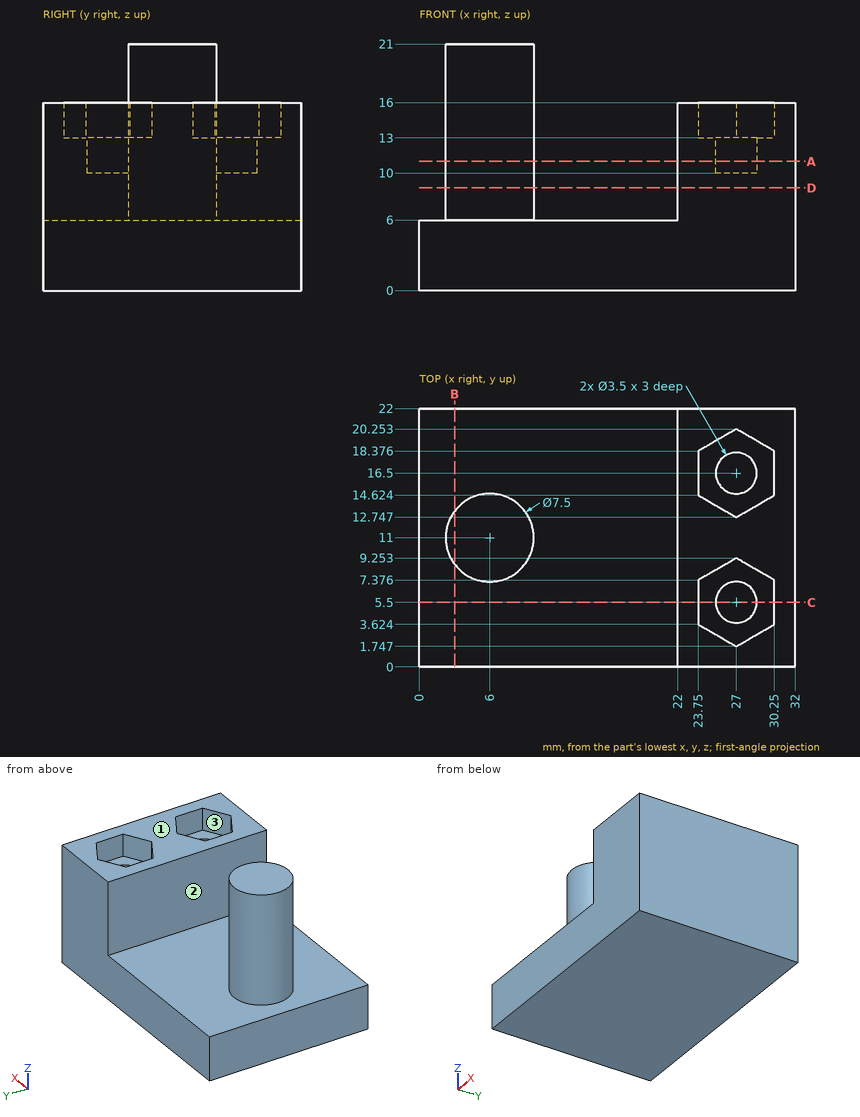
Geometry: see drawing. Coordinates: mm, zero at the bounding-box minimum. A direction names the side the tool comes from. Give positions to 0.01 mm unless a question says otherwise; leave off trailing zeros. Loops run counter-clockwise (first coordinate to the right, second up) from the corner with the lowest first, then second, coordinate; pieces in that order, holes last. Notation, with made-up numbers: (-8.75, 23.5) - (11.25, 23.5) arc R19 ccw to (11.25, 54.5) - close; hole circle Ø11 at (75.25, 71). An arc over 180 degrees is marked (long way). One line per question, with ' | ' between items. Start each with the question number.
(1) Section query D-D on z = 8.75. Return loops of the section in (x, y), then the cut area to 3 significant figures.
(2) Section query C-C on y = 5.5. Return loops of the section in (x, z), then the cut area to 3 significant figures.
(3) Contact query for flat-ended pins moving along their axis: pin 1 (3 mm diameter, centred on y = 12, z = 9.5, fed in from -X); pin 2 (4 mm diameter, centred on x = 27, y = 17, fed in from +Z); pin 3 (12 mm diameter, centred on x = 25.5, z = 15.5, fed in from -Y); pin 4 (8 mm diameter, centred on x = 26, y = 13.5, fed in from +Z). Output: stop coordinate, or through.
(4) Ray query, line 1 (Y direction, x = 27, z = 12.2); line 2 (X direction, y = 8, z = 15.25); line 3 (Z direction, x = 7.5, y = 5.25). Return the intervals inside material, ascending. Write a range as from..to.
(5) Section query A-A on z = 11. Return loops of the section in (x, y), then the cut area to 3 significant figures.
(6) Section query B-B on x = 3. Return loops of the section in (y, z).
(7) Reachability of the marked faces 1, 2 and 3 from +Z, -Z, +X, -X, +Y, -Y: full face, straight path, thin tool, end or side. Return the list, or none.
The answers:
1) outline: circle Ø7.5 at (6, 11); (22, 0) - (32, 0) - (32, 22) - (22, 22) - close | area: 264 mm2
2) outline: (0, 0) - (32, 0) - (32, 16) - (30.25, 16) - (30.25, 13) - (28.75, 13) - (28.75, 10) - (25.25, 10) - (25.25, 13) - (23.75, 13) - (23.75, 16) - (22, 16) - (22, 6) - (0, 6) - close | area: 262 mm2
3) pin 1: x = 2.25 | pin 2: z = 13 | pin 3: y = 0 | pin 4: z = 16
4) line 1: 0..3.75, 7.25..14.75, 18.25..22 | line 2: 3.75..8.25, 22..24.83, 29.17..32 | line 3: 0..6
5) outline: circle Ø7.5 at (6, 11); (22, 0) - (32, 0) - (32, 22) - (22, 22) - close; hole circle Ø3.5 at (27, 5.5); hole circle Ø3.5 at (27, 16.5) | area: 245 mm2
6) outline: (0, 0) - (22, 0) - (22, 6) - (13.25, 6) - (13.25, 21) - (8.75, 21) - (8.75, 6) - (0, 6) - close
7) face 1: +Z, +X, +Y, -Y | face 2: +Z, +Y, -Y | face 3: +Z
